Geometry: see drawing. Coordinates: mm, zero at the bounding-box minimum. A direction names the side the tool comes from. Coordinates: 2 decimals unless noted, no trailing zeros. Order: outer loops, then holes, each group sorted by start corner. A loop starts at its lowest first (then second) coordinate and runs counter-clockwise, first axis right, second up.
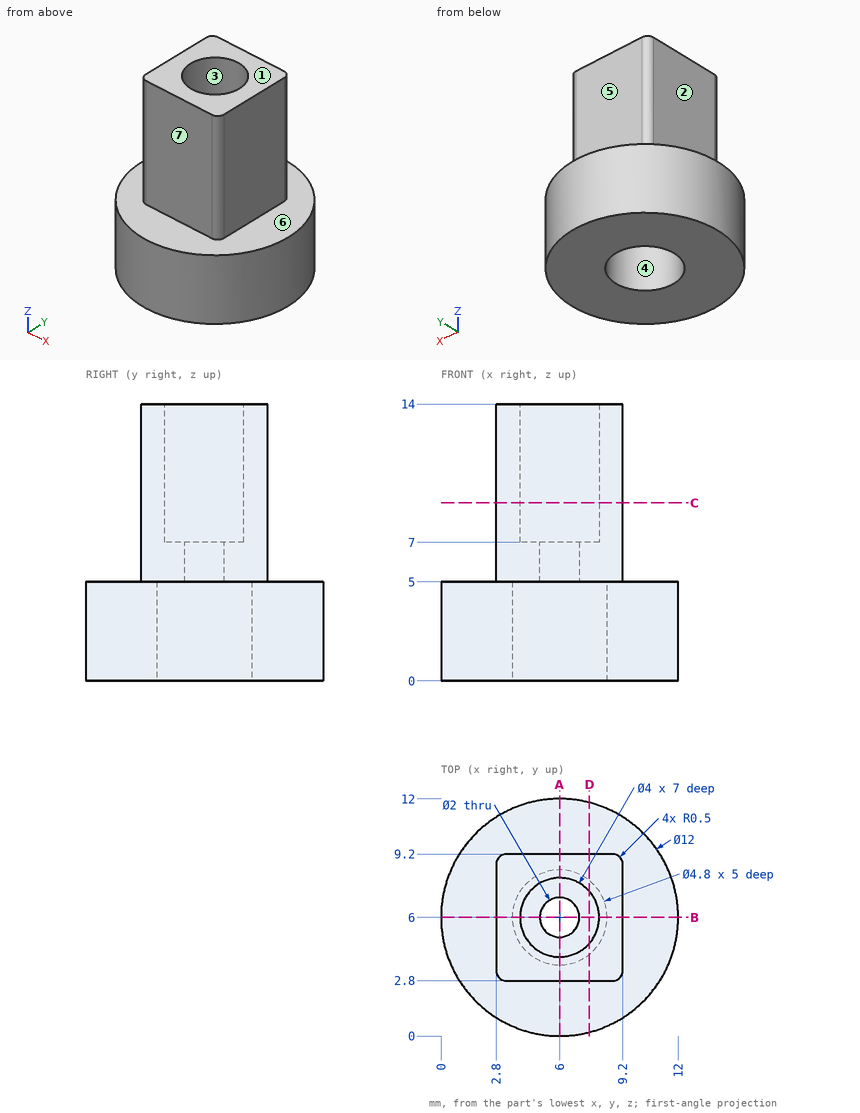
Q1. Set-up query: the marked faces 4, 5, 6 and 7. Return all of +Z, -Z, +X, -X, +Y, -Y with unobstructed straight access to the full face (end or side cutting, diameter ignored); none if empty.
Solutions:
face 4: -Z
face 5: +Z, +X, -X, +Y
face 6: +Z
face 7: +Z, +X, -X, -Y
Q2. Pin query (flat end, axial travel): P1, Ø1, axis at y = 5, z = 3, coming from the +X side; P2, Ø1.6, axis at y = 5, z = 10.5, coming from the -X side; P3, Ø1, axis at x = 11, z = 1.5, coming from the +Y side; P4, Ø3, axis at x = 6, y = 5, coming from the +Z side. Return the tip coordinate at first contact, or that it passes through.
Solutions:
P1: stops at x = 11.98
P2: stops at x = 2.8
P3: stops at y = 9.97
P4: stops at z = 14
Q3. Section query C-C on z = 9. Output: boundary loops of the cut face in (x, y), plus the area to 3 significant figures.
Solutions:
outline: (2.8, 3.3) arc R0.5 ccw to (3.3, 2.8) - (8.7, 2.8) arc R0.5 ccw to (9.2, 3.3) - (9.2, 8.7) arc R0.5 ccw to (8.7, 9.2) - (3.3, 9.2) arc R0.5 ccw to (2.8, 8.7) - close; hole circle Ø4 at (6, 6)
area: 28.2 mm2
Q4. Material intervals for line 1 along Y through (x, z) = (6, 2.6); line 2 along Y through (x, z) = (6, 10.5); line 3 along X through (y, z) = (3.25, 7), sorted ascending.
Solutions:
line 1: y = 0 to 3.6, 8.4 to 12
line 2: y = 2.8 to 4, 8 to 9.2
line 3: x = 2.8 to 9.2
Q5. Section query D-D on x = 7.5. Output: boundary loops of the cut face in (y, z), plus the area to 3 significant figures.
Solutions:
outline: (0.19, 0) - (4.13, 0) - (4.13, 5) - (7.87, 5) - (7.87, 0) - (11.81, 0) - (11.81, 5) - (9.2, 5) - (9.2, 14) - (7.32, 14) - (7.32, 7) - (4.68, 7) - (4.68, 14) - (2.8, 14) - (2.8, 5) - (0.19, 5) - close
area: 78.4 mm2
Q6. Pull-direction query (X, two-part tool) for the marked faces 1, 2 and 3; classes: pulls with the +X half, pulls with the -X half, needs draft (parallel to the pull), parting line crosses it, or undercut.
Solutions:
face 1: needs draft
face 2: pulls with the -X half
face 3: undercut
Q7. Section query A-A on x = 6. Output: boundary loops of the cut face in (y, z), plus the area to 3 significant figures.
Solutions:
outline: (0, 0) - (3.6, 0) - (3.6, 5) - (5, 5) - (5, 7) - (4, 7) - (4, 14) - (2.8, 14) - (2.8, 5) - (0, 5) - close; (7, 5) - (8.4, 5) - (8.4, 0) - (12, 0) - (12, 5) - (9.2, 5) - (9.2, 14) - (8, 14) - (8, 7) - (7, 7) - close
area: 61.6 mm2
